Can you work these out from the model? Positions are in its coordinate system, mm. A direction names the side the tool comes from. Give positions to 0.01 mm unless a question says otherwise; leave off trailing zeros. Loops run counter-clockwise (first coordinate to the right, second up) from the corner with the lowest first, then second, coordinate; pieces in that order, holes last. Notation, with made-up numbers: M -0.5,26.5 L 32.5,26.5 A16 cw 32.5,56.5 Z; hole C -1.5,-24 d4. An arc over 180 degrees is marked long. Answer as a JSON object with one key per item and string values.
```python
from build123d import *

# Parameters (mm, degrees)
F0_R     = 1.2
F1_DEPTH = 6.4
F2_W     = 0.5
F2_H     = 3.2
F3_DEPTH = 2
F4_W     = 0.3
F4_H     = 4
F5_DEPTH = 2


with BuildPart() as f1:
    # F0 (on Front) → F1 (new body)
    with BuildSketch(Plane.XZ):
        with BuildLine():
            ThreePointArc((0, 0.5), (0.146447, 0.146447), (0.5, 0))
            Line((0.5, 0), (3.35, 0))
            Line((3.35, 0), (3.75, -0.4))
            Line((3.75, -0.4), (6.75, -0.4))
            Line((6.75, -0.4), (7.15, 0))
            Line((7.15, 0), (12.85, 0))
            Line((12.85, 0), (13.25, -0.4))
            Line((13.25, -0.4), (16.25, -0.4))
            Line((16.25, -0.4), (16.65, 0))
            Line((16.65, 0), (19.5, 0))
            ThreePointArc((19.5, 0), (19.853553, 0.146447), (20, 0.5))
            Line((20, 0.5), (20, 8.5))
            ThreePointArc((20, 8.5), (19.707107, 9.207107), (19, 9.5))
            Line((19, 9.5), (10.7, 9.5))
            Line((10.7, 9.5), (10, 10.2))
            Line((10, 10.2), (1, 10.2))
            ThreePointArc((1, 10.2), (0.292893, 9.907107), (0, 9.2))
            Line((0, 9.2), (0, 0.5))
        make_face()
        with Locations((5.25, 2.5)):
            Circle(F0_R, mode=Mode.SUBTRACT)
        with Locations((14.75, 2.5)):
            Circle(F0_R, mode=Mode.SUBTRACT)
    extrude(amount=F1_DEPTH)

    # F2 (on face) → F3 (cut)
    with BuildSketch(Plane(origin=(0, 0, 0), x_dir=(1, 0, 0), z_dir=(0, 0, -1))):
        with Locations((1.9, 3.2)):
            Rectangle(F2_W, F2_H)
        with Locations((10.7, 3.2)):
            Rectangle(F2_W, F2_H)
        with Locations((18, 3.2)):
            Rectangle(F2_W, F2_H)
    extrude(amount=-F3_DEPTH, mode=Mode.SUBTRACT)

    # F4 (on face) → F5 (cut)
    with BuildSketch(Plane.XY.offset(10.2)):
        with Locations((3.05, -3.2)):
            Rectangle(F4_W, F4_H)
    extrude(amount=-F5_DEPTH, mode=Mode.SUBTRACT)


solid = f1.part
```
1) Please list where these lines run through material, in increasing order: line 1 along Z through (x, y) = (14.75, -3); line 2 along X through (y, z) = (-3.5, 1.25); line 3 along X through (y, z) = (-4.25, 3.5). Write a range as from..to.
Answer list:
{"line 1": "-0.4..1.3, 3.7..9.5", "line 2": "0..1.65, 2.15..10.45, 10.95..17.75, 18.25..20", "line 3": "0..4.59, 5.91..14.09, 15.41..20"}
2) Suppose I cut it at A-A, the plane z = 1.75. Write out the boundary of the cut face in (x, y).
Answer list:
{"outline": "M 0,-6.4 L 4.31,-6.4 L 4.31,0 L 0,0 Z; M 6.19,-6.4 L 13.81,-6.4 L 13.81,0 L 6.19,0 Z; M 15.69,-6.4 L 20,-6.4 L 20,0 L 15.69,0 Z; hole M 1.65,-4.8 L 2.15,-4.8 L 2.15,-1.6 L 1.65,-1.6 Z; hole M 10.45,-4.8 L 10.95,-4.8 L 10.95,-1.6 L 10.45,-1.6 Z; hole M 17.75,-4.8 L 18.25,-4.8 L 18.25,-1.6 L 17.75,-1.6 Z"}
3) Will these pins go through, and if not, where does the flat tip stop? pin 1 Ø3 at (x, y) = (18.5, -3) entering from -Z; pin 2 Ø1.9 at (x, z) = (14.75, 2.5) entering from -Y.
Answer list:
{"pin 1": "z = 0", "pin 2": "through"}
4) Suppose I cut it at D-D, the plane x = 5.25. Write out the boundary of the cut face in (y, z), and give its area (3 significant figures).
Answer list:
{"outline": "M -6.4,-0.4 L 0,-0.4 L 0,1.3 L -6.4,1.3 Z; M -6.4,3.7 L 0,3.7 L 0,10.2 L -6.4,10.2 Z", "area": "52.5 mm^2"}
5) For faces 1 (the flat face through (3, -3, 0)), 2 (the flat face through (17, -3, 0)), 3 (the flat face through (18.25, -3, 1)), which set-ups out of +Z, -Z, +X, -X, +Y, -Y let a thin tool reach every point of the face, with its end or its side?
Answer list:
{"face 1": "-Z, -X, +Y, -Y", "face 2": "-Z, +X, +Y, -Y", "face 3": "-Z"}
6) Suppose I cut it at C-C, the plane y = -5. Write out the boundary of the cut face in (x, z).
Answer list:
{"outline": "M 0,0.5 A0.5 ccw 0.5,0 L 3.35,0 L 3.75,-0.4 L 6.75,-0.4 L 7.15,0 L 12.85,0 L 13.25,-0.4 L 16.25,-0.4 L 16.65,0 L 19.5,0 A0.5 ccw 20,0.5 L 20,8.5 A1 ccw 19,9.5 L 10.7,9.5 L 10,10.2 L 3.2,10.2 L 3.2,8.2 L 2.9,8.2 L 2.9,10.2 L 1,10.2 A1 ccw 0,9.2 Z; hole C 5.25,2.5 d2.4; hole C 14.75,2.5 d2.4"}
7) Suppose I cut it at B-B, the plane x = 14.75. Write out the boundary of the cut face in (y, z).
Answer list:
{"outline": "M -6.4,-0.4 L 0,-0.4 L 0,1.3 L -6.4,1.3 Z; M -6.4,3.7 L 0,3.7 L 0,9.5 L -6.4,9.5 Z"}
8) If we mould it in two halves opening along Y, with no side actions, what happens to faces 4 (the flat face through (10, -6.4, 5)), 5 (the flat face through (2.9, -3, 9)), 6 (the flat face through (20, -3, 4))? For each: +Y half, -Y half, draft (parallel to the pull), parting line (faces both ways), or undercut.
Answer list:
{"face 4": "-Y half", "face 5": "undercut", "face 6": "draft"}
